```python
from build123d import *

# Parameters (mm, degrees)
SZKIC1_W                    = 12
SZKIC1_H                    = 20
DODANIE_WYCI_GNI_CIE1_DEPTH = 85
SZKIC2_R                    = 1.5
WYTNIJ_WYCI_GNI_CIE1_DEPTH  = 10
SZKIC4_R                    = 6.5
WYTNIJ_WYCI_GNI_CIE2_DEPTH  = 5
SZKIC5_R                    = 4.5
WYTNIJ_WYCI_GNI_CIE3_DEPTH  = 87.423376467
SZKIC6_R                    = 1.1
WYTNIJ_WYCI_GNI_CIE4_DEPTH  = 87.423376467
SFAZOWANIE1_SIZE            = 0.5
SZKIC7_R                    = 1.1
WYTNIJ_WYCI_GNI_CIE5_DEPTH  = 87.423376467
SFAZOWANIE2_SIZE            = 0.5
ZAOKR_GLENIE1_R             = 5
WYTNIJ_WYCI_GNI_CIE6_DEPTH  = 87.423376493
ZAOKR_GLENIE2_R             = 1


with BuildPart() as part:
    # Szkic1 → Dodanie-wyciągnięcie1 (new body)
    with BuildSketch(Plane.XY):
        Rectangle(SZKIC1_W, SZKIC1_H)
    extrude(amount=DODANIE_WYCI_GNI_CIE1_DEPTH)

    # Szkic2 → Wytnij-wyciągnięcie1 (cut)
    with BuildSketch(Plane.XY.offset(85)):
        with Locations((-3, 7)):
            Circle(SZKIC2_R)
        with Locations((3, -7)):
            Circle(SZKIC2_R)
    extrude(amount=-WYTNIJ_WYCI_GNI_CIE1_DEPTH, mode=Mode.SUBTRACT)

    # Szkic4 → Wytnij-wyciągnięcie2 (cut)
    with BuildSketch(Plane(origin=(6, 0, 0), x_dir=(0, 0, -1), z_dir=(1, 0, 0))):
        with Locations((-15, 0)):
            Circle(SZKIC4_R)
    extrude(amount=-WYTNIJ_WYCI_GNI_CIE2_DEPTH, mode=Mode.SUBTRACT)

    # Szkic5 → Wytnij-wyciągnięcie3 (cut, through all)
    with BuildSketch(Plane.ZY.offset(6)):
        with Locations((15, 0)):
            Circle(SZKIC5_R)
    extrude(amount=-WYTNIJ_WYCI_GNI_CIE3_DEPTH, mode=Mode.SUBTRACT)

    # Szkic6 → Wytnij-wyciągnięcie4 (cut, through all)
    with BuildSketch(Plane.ZY.offset(6)):
        with Locations((34.05, 0)):
            Circle(SZKIC6_R)
    extrude(amount=-WYTNIJ_WYCI_GNI_CIE4_DEPTH, mode=Mode.SUBTRACT)

    # Sfazowanie1
    sfazowanie1_edges = [part.edges().sort_by_distance(p)[0] for p in [
        (6, 0, 32.95),
    ]]
    chamfer(sfazowanie1_edges, length=SFAZOWANIE1_SIZE)

    # Szkic7 → Wytnij-wyciągnięcie5 (cut, through all)
    with BuildSketch(Plane.ZY.offset(6)):
        with Locations((6.25, 0)):
            Circle(SZKIC7_R)
    extrude(amount=-WYTNIJ_WYCI_GNI_CIE5_DEPTH, mode=Mode.SUBTRACT)

    # Sfazowanie2
    sfazowanie2_edges = [part.edges().sort_by_distance(p)[0] for p in [
        (6, 0, 5.15),
    ]]
    chamfer(sfazowanie2_edges, length=SFAZOWANIE2_SIZE)

    # Zaokrąglenie1
    # the kernel refuses this fillet: 5 mm, written as the material it takes off along each edge
    with BuildSketch(Plane(origin=(-18.5, -10, 0), x_dir=(0, 0, 1), z_dir=(1, 0, 0))) as zaokr_glenie1_piece_1:
        with BuildLine():
            CenterArc((ZAOKR_GLENIE1_R, -ZAOKR_GLENIE1_R), ZAOKR_GLENIE1_R, 90, 90)
            Line((0, -ZAOKR_GLENIE1_R), (0, 0))
            Line((0, 0), (ZAOKR_GLENIE1_R, 0))
        make_face()
    extrude(amount=37, mode=Mode.SUBTRACT)
    with BuildSketch(Plane(origin=(18.5, 10, 0), x_dir=(0, -1, 0), z_dir=(-1, 0, 0))) as zaokr_glenie1_piece_2:
        with BuildLine():
            CenterArc((ZAOKR_GLENIE1_R, ZAOKR_GLENIE1_R), ZAOKR_GLENIE1_R, 180, 90)
            Line((0, ZAOKR_GLENIE1_R), (0, 0))
            Line((0, 0), (ZAOKR_GLENIE1_R, 0))
        make_face()
    extrude(amount=37, mode=Mode.SUBTRACT)
    with BuildSketch(Plane(origin=(6, -22.5, 0), x_dir=(0, 0, 1), z_dir=(0, 1, 0))) as zaokr_glenie1_piece_3:
        with BuildLine():
            CenterArc((ZAOKR_GLENIE1_R, -ZAOKR_GLENIE1_R), ZAOKR_GLENIE1_R, 90, 90)
            Line((0, -ZAOKR_GLENIE1_R), (0, 0))
            Line((0, 0), (ZAOKR_GLENIE1_R, 0))
        make_face()
    extrude(amount=45, mode=Mode.SUBTRACT)

    # Szkic8 → Wytnij-wyciągnięcie6 (cut, through all)
    with BuildSketch(Plane.ZY.offset(6)):
        with BuildLine():
            Line((37.668037351, -4), (37.668037351, 4))
            ThreePointArc((37.668037351, 4), (39.668037351, 6), (41.668037351, 4))
            Line((41.668037351, 4), (41.668037351, -4))
            ThreePointArc((41.668037351, -4), (39.668037351, -6), (37.668037351, -4))
        make_face()
    extrude(amount=-WYTNIJ_WYCI_GNI_CIE6_DEPTH, mode=Mode.SUBTRACT)

    # Zaokrąglenie2
    zaokr_glenie2_edges = [part.edges().sort_by_distance(p)[0] for p in [
        (6, -6, 39.668037351),
        (6, 0, 37.668037351),
        (6, 6, 39.668037351),
        (6, 0, 41.668037351),
        (-6, -6, 39.668037351),
        (-6, 0, 41.668037351),
        (-6, 6, 39.668037351),
        (-6, 0, 37.668037351),
    ]]
    fillet(zaokr_glenie2_edges, radius=ZAOKR_GLENIE2_R)


solid = part.part
```
The model under review builds one solid part; all positions refer to its coordinate system, in mm. A direction names the side the tool comes from. Round coordinates to 2 decimals unless told otherwise and drop trailing zeros. Loops run counter-clockwise (first coordinate to the right, second up) from the corner with the lowest first, then second, coordinate; pieces in that order, holes last. Notation, with made-up numbers: M 17.25,-31.5 L 39.25,-31.5 A21 ccw 39.25,-27.5 Z; hole C -5.75,-16 d3. An arc over 180 degrees is marked long. Put each result on its own line as item: value.
Q1. Machinability: for faces 1 (the flat face through (-3, 7, 75)), 2 (the cylindrical face through (3.535, 0.286, 21.494)), 3 (the flat face through (0, 0, 41.668)), which of the approach directions +Z, -Z, +X, -X, +Y, -Y give a long, thin tool a straight path to every point of the face, cutting with its end or side? Answer none if there is none.
Result set:
face 1: +Z
face 2: +X
face 3: +X, -X
Q2. For pin 1 (3 mm diameter, centred on y = 0, z = 34.05, fed in from +X); pin 2 (1.8 mm diameter, centred on x = -3, y = 7, fed in from -Z); pin 3 (7 mm diameter, centred on y = 0, z = 15, fed in from +X); pin 4 (6.5 mm diameter, centred on y = 1.5, z = 14, fed in from +X), all flat-tipped, find the tip position at first contact; note any pin that passes through.
Result set:
pin 1: stops at x = 5.9
pin 2: stops at z = 0.12
pin 3: passes through
pin 4: stops at x = 1
Q3. Mouldability with a two-part tool opening along Y and no side actions: class faces 4 (the cylindrical face through (-1, 9, 2)), 5 (the cylindrical face through (-2.549, 0.198, 10.504)), 6 (the cylindrical face through (-0.1, 6, 39.6)), 7 (the flat face through (-3, 0, 0)) as released by +Y, released by -Y, zero draft, split by the parting line, or undercut.
Result set:
face 4: released by +Y
face 5: undercut
face 6: undercut
face 7: zero draft
Q4. To check wall thickness, follow L1, parallel to Y at x = -2, z = 6.25; L2, parallel to Y at x = 3, z = 82.25; L3, parallel to Z at x = -3.75, y = 1.75. State the ranges of each line that lie inside material, in increasing order.
Result set:
L1: y = -10 to -1.1, 1.1 to 10
L2: y = -10 to -8.5, -5.5 to 10
L3: z = 0 to 10.85, 19.15 to 37.67, 41.67 to 85
Q5. Consider section C-C, the plane x = 3. Give the boundary of the cut face in (y, z).
Result set:
outline: M -10,5 A5 ccw -7,0.42 L 7,0.42 A5 ccw 10,5 L 10,85 L -5.5,85 L -5.5,75 L -8.5,75 L -8.5,85 L -10,85 Z; hole C 0,15 d13; hole M -4,37.67 L 4,37.67 A2 ccw 4,41.67 L -4,41.67 A2 ccw Z; hole C 0,6.25 d2.2; hole C 0,34.05 d2.2
Q6. Consider section B-B, the plane x = -3. Give the boundary of the cut face in (y, z).
Result set:
outline: M -10,5 A5 ccw -5,0 L 5,0 A5 ccw 10,5 L 10,85 L 8.5,85 L 8.5,75 L 5.5,75 L 5.5,85 L -10,85 Z; hole C 0,15 d9; hole M -4,37.67 L 4,37.67 A2 ccw 4,41.67 L -4,41.67 A2 ccw Z; hole C 0,6.25 d2.2; hole C 0,34.05 d2.2
Q7. Consider section A-A, the plane z = 15. Give the boundary of the cut face in (x, y).
Result set:
outline: M -6,-10 L 6,-10 L 6,-6.5 L 1,-6.5 L 1,-4.5 L -6,-4.5 Z; M -6,4.5 L 1,4.5 L 1,6.5 L 6,6.5 L 6,10 L -6,10 Z
